For this review, use the dimensioned drawing (mm, ordinates from the lowest corner) and the shaded views. A direction names the side the tool comes from. Round coordinates to 2 decimals unless told otherwise and drop trailing zeros. Loops run counter-clockwise (first coordinate to the right, second up) from the corner with the lowest first, then second, coordinate; pieces in that order, holes last. Notation, with made-up numbers: (0, 83) - (30, 83) arc R22 cw to (30, 116) - close; hole circle Ø5 at (71.5, -11.5). An arc over 180 degrees is marked (long way). Return JSON: item names as keys, results as strings. Group by question number.
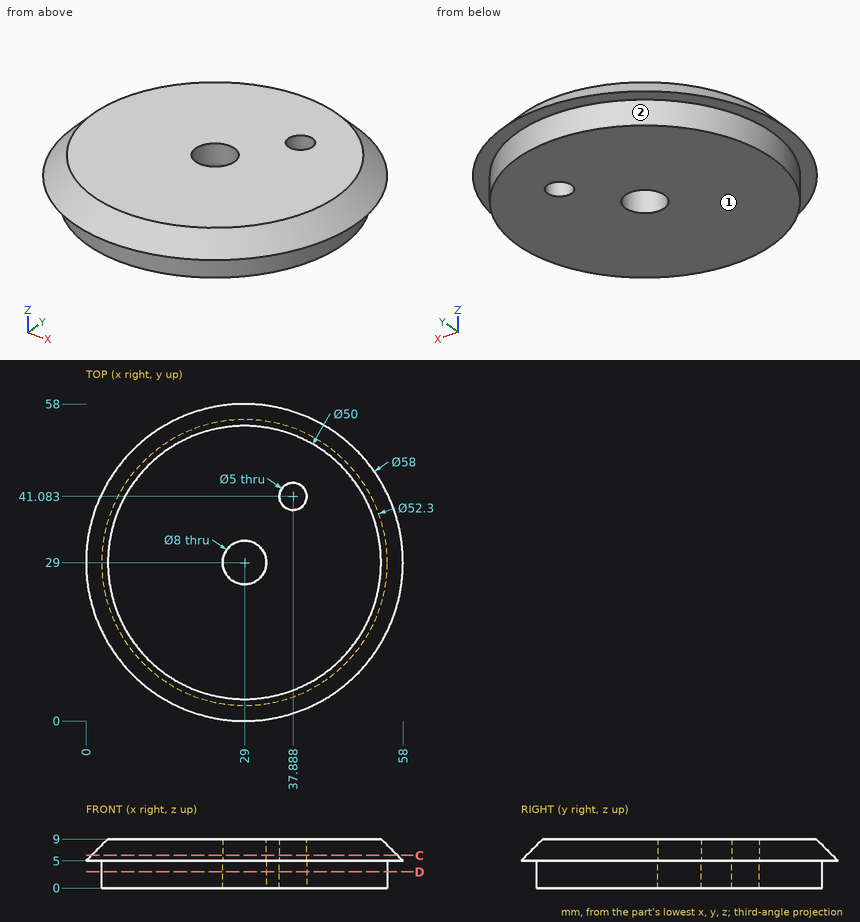
Q1. Tool access review of the marked faces 1 and 2: name each direction out of +Z, -Z, +X, -X, +Y, -Y from which nothing blocks a thin tool from reaching the whole face with its end or side.
Q2. For line 1 (Y direction, x = 29, z = 1.4); line 2 (X direction, y = 30.5, z = 3.5); line 3 (X direction, y = 42.5, z = 3.5) (1 decimal), list the stretches that pass through material, from the lowest coordinate up.
Q3. Add section D-D, the plane z = 3. State the section outline as (x, y) points.
Q4. Insertion check: pin 1 Ø8 at (x, y) = (24, 9) entering from -Z; pin 2 Ø1 at (y, z) = (37, 1.5) entering from -X; pin 3 Ø6.5 at (x, y) = (29, 29) entering from -Z; pin 4 Ø2 at (y, z) = (39.5, 6.5) entering from +X (1 decimal). Each pin has a flat end and moves straight along its axis. Give the tip position at first contact, or say it passes through.
Q5. Add section C-C, the plane z = 6. State the section outline as (x, y) points, plus the area to 3 significant figures.
Evaluation:
{
 "1": {"face 1": "-Z, +X, -X, +Y, -Y", "face 2": "-Z"},
 "2": {"line 1": "2.85 to 25, 33 to 55.15", "line 2": "2.89 to 25.29, 32.71 to 55.11", "line 3": "6.6 to 35.8, 39.9 to 51.4"},
 "3": {"outline": "circle Ø52.3 at (29, 29); hole circle Ø8 at (29, 29); hole circle Ø5 at (37.89, 41.08)"},
 "4": {"pin 1": "z = 0", "pin 2": "x = 3.95", "pin 3": "through", "pin 4": "x = 55.6"},
 "5": {"outline": "circle Ø56 at (29, 29); hole circle Ø8 at (29, 29); hole circle Ø5 at (37.89, 41.08)", "area": "2,390 mm²"}
}
